Design review of the part built by this model. Coordinates are the model's own, in mm. A direction names the side the tool comes from. Give positions to 0.01 mm unless a question says otherwise; leave off trailing zeros. Order: outer loops, then holes, each group sorted by start corner. A loop starts at its lowest first (then second) coordinate and runs counter-clockwise, first axis right, second up. Notation, with made-up numbers: (-4, 53) -> (28, 53) arc R20 cw to (28, 64) -> close; hole circle Ø6 at (61, 45.5). An arc over 180 degrees is marked (long way). Return JSON: item names as keys, results as strings.
```python
from build123d import *

# Parameters (mm, degrees)
F0_W     = 10
F0_H     = 60
F0_R     = 1.5
F1_DEPTH = 2.5
F2_DEPTH = 5
F3_R     = 4.99999


# Not quite as in the source:
# - a fillet or chamfer is up to 0.001 mm smaller than in the source, because OpenCascade refuses the exact size


with BuildPart() as f1:
    # F0 (on Top) → F1 (new body, symmetric)
    with BuildSketch(Plane.XY):
        with Locations((-32.8091010451, 20.9925968945)):
            Rectangle(F0_W, F0_H)
        with Locations((-32.8091010451, -3.8919287648)):
            Circle(F0_R, mode=Mode.SUBTRACT)
        with Locations((-32.8091010451, 49.3113994598)):
            Circle(F0_R, mode=Mode.SUBTRACT)
    extrude(amount=F1_DEPTH, both=True)

    # F0 (on Top) → F2 (join)
    with BuildSketch(Plane.XY):
        with Locations((-32.8091010451, 49.3113994598)):
            Circle(F0_R)
        with Locations((-32.8091010451, -3.8919287648)):
            Circle(F0_R)
    extrude(amount=-F2_DEPTH)

    # F3 (radius 5 in the source; OpenCascade refuses exactly that, so slightly less here)
    f3_edges = [f1.edges().sort_by_distance(p)[0] for p in [
        (-27.809101, 50.992597, 0),
        (-37.809101, 50.992597, 0),
        (-27.809101, -9.007403, 0),
        (-37.809101, -9.007403, 0),
    ]]
    fillet(f3_edges, radius=F3_R)


solid = f1.part
```
Item 1: Wall thickness on L1, parallel to Y at x = -33, z = 2.25; L2, parallel to Z at x = -37, y = 16.5; L3, parallel to Y at x = -32.5, z = -3: over which ranges is each line inside the solid? List them lowest first. Write a range as [from, to].
Result set:
{"L1": "y = [-9, -5.38], [-2.4, 47.82], [50.8, 50.99]", "L2": "z = [-2.5, 2.5]", "L3": "y = [-5.36, -2.42], [47.84, 50.78]"}
Item 2: For pin 1 (1.8 mm diameter, centred on x = -32.81, y = -3.89, fed in from +Z); pin 2 (6 mm diameter, centred on x = -32.5, y = 19, fed in from -Z); pin 3 (2 mm diameter, centred on x = -29, z = 1, fed in from -Y), all flat-tipped, find the tip position at first contact; note any pin that passes through.
Result set:
{"pin 1": "stops at z = 0", "pin 2": "stops at z = -2.5", "pin 3": "stops at y = -8.14"}
Item 3: Add section B-B (x = -33.5). Give the boundary of the cut face in (y, z).
Result set:
{"outline": "(-8.96, -2.5) -> (-5.22, -2.5) -> (-5.22, -5) -> (-2.56, -5) -> (-2.56, -2.5) -> (47.98, -2.5) -> (47.98, -5) -> (50.64, -5) -> (50.64, -2.5) -> (50.94, -2.5) -> (50.94, 2.5) -> (50.64, 2.5) -> (50.64, 0) -> (47.98, 0) -> (47.98, 2.5) -> (-2.56, 2.5) -> (-2.56, 0) -> (-5.22, 0) -> (-5.22, 2.5) -> (-8.96, 2.5) -> close"}
Item 4: Machinability: for faces 1 (the face through (-36.38, 49.49, -0.04)), 2 (the face through (-31.378, 49.762, -3.732)), 3 (the face through (-33, -4, 0)), which of the approach directions +Z, -Z, +X, -X, +Y, -Y give a long, thin tool a straight path to every point of the face, cutting with its end or side? Answer none if there is none.
Result set:
{"face 1": "+Z, -Z, -X, +Y", "face 2": "-Z", "face 3": "+Z"}
Item 5: Add section D-D (z = 1.75). Give the number of separate pieces and of enclosed holes in the cut face, plus the area to 3 significant figures.
Result set:
{"separate pieces": "1", "enclosed holes": "2", "area": "564 mm^2"}
Item 6: Add section C-C (y = 18). Give the boundary of the cut face in (x, z), plus the area to 3 significant figures.
Result set:
{"outline": "(-37.81, -2.5) -> (-27.81, -2.5) -> (-27.81, 2.5) -> (-37.81, 2.5) -> close", "area": "50.0 mm^2"}
Item 7: Mouldability with a two-part tool opening along X and no side actions: class faces 4 (the face through (-27.809, 21, 0)), 5 (the face through (-31.38, -3.44, 1.23)), 6 (the face through (-33, 21, -2.5)) as released by +X, released by -X, zero draft, split by the parting line, or undercut.
Result set:
{"face 4": "released by +X", "face 5": "undercut", "face 6": "zero draft"}
